Geometry check sheet. Reference: the model listing, model coordinates, mm. A direction names the side the tool comes from. Round coordinates to 2 decimals unless told otherwise and drop trailing zeros. Write each loop counter-clockwise with the first axis right and the second up, starting at its lowest first coordinate (ties: lowest second). Pieces come first, ordered by that corner, then holes. Notation, with made-up numbers: (47, -2.75) - (66, -2.75) arc R28 ccw to (66, 18.25) - close; hole circle Ø11 at (62, -39). An arc over 180 degrees is marked (long way). Return JSON: item names as keys, results as strings.
```python
from build123d import *

# Parameters (mm, degrees)
SKETCH1_W                = 15.24
SKETCH1_H                = 30.9118
BOSS_EXTRUDE1_DEPTH      = 31.115
BOSS_EXTRUDE2_DEPTH      = 6.9215
BOSS_EXTRUDE2_DEPTH_BACK = 37.9095
SKETCH2_W                = 15.24
SKETCH2_H                = 6.096
SKETCH3_R                = 5.2705
BOSS_EXTRUDE3_DEPTH      = 3.9624
SKETCH4_R                = 6.3119
BOSS_EXTRUDE4_DEPTH      = 2.5019
CUT_EXTRUDE1_REACH       = 50.11
SKETCH8_R                = 1.5621
CUT_EXTRUDE2_REACH       = 50.11
SKETCH9_R                = 1.5621
SKETCH10_R               = 3.99415
BOSS_EXTRUDE5_DEPTH      = 2.0828
SKETCH13_R               = 1.5875
CUT_EXTRUDE3_DEPTH       = 2.54


with BuildPart() as part:
    # Sketch1 → Boss-Extrude1 (new body)
    with BuildSketch(Plane(origin=(0, 0, 0), x_dir=(1, 0, 0), z_dir=(0, 1, 0))):
        with Locations((7.62, 15.4559)):
            Rectangle(SKETCH1_W, SKETCH1_H)
    extrude(amount=BOSS_EXTRUDE1_DEPTH)

    # Sketch2 → Boss-Extrude2 (add, two sides: drawn at the far end of the back side and taken through both)
    with BuildSketch(Plane.XY.offset(-BOSS_EXTRUDE2_DEPTH_BACK)):
        with Locations((7.62, 22.352)):
            Rectangle(SKETCH2_W, SKETCH2_H)
    extrude(amount=BOSS_EXTRUDE2_DEPTH + BOSS_EXTRUDE2_DEPTH_BACK)

    # Sketch3 → Boss-Extrude3 (add)
    with BuildSketch(Plane(origin=(0, 0, -30.9118), x_dir=(-1, 0, 0), z_dir=(0, 0, -1))):
        with Locations(Location((-7.62, 8.2804, 0), (0, 0, 180))):
            Circle(SKETCH3_R)
    extrude(amount=BOSS_EXTRUDE3_DEPTH)

    # Sketch4 → Boss-Extrude4 (add)
    with BuildSketch(Plane(origin=(0, 31.115, 0), x_dir=(1, 0, 0), z_dir=(0, 1, 0))):
        with Locations(Location((7.62, 24.2951, 0), (0, 0, 90))):
            Circle(SKETCH4_R)
    extrude(amount=BOSS_EXTRUDE4_DEPTH)

    # Sketch8 → Cut-Extrude1 (cut, up to next)
    with BuildSketch(Plane(origin=(0, 25.4, 0), x_dir=(1, 0, 0), z_dir=(0, 1, 0)), mode=Mode.PRIVATE) as cut_extrude1_sk1:
        with Locations(Location((7.62, -3.46075, 0), (0, 0, 270))):
            Circle(SKETCH8_R)
    cut_extrude1_tool1 = extrude(cut_extrude1_sk1.sketch, amount=-CUT_EXTRUDE1_REACH, mode=Mode.PRIVATE) & part.part
    add(cut_extrude1_tool1.solids().sort_by_distance((7.62, 25.4, 3.46075))[0], mode=Mode.SUBTRACT)

    # Sketch9 → Cut-Extrude2 (cut, up to next)
    with BuildSketch(Plane(origin=(0, 25.4, 0), x_dir=(1, 0, 0), z_dir=(0, 1, 0)), mode=Mode.PRIVATE) as cut_extrude2_sk1:
        with Locations(Location((7.62, 34.41065, 0), (0, 0, 270))):
            Circle(SKETCH9_R)
    cut_extrude2_tool1 = extrude(cut_extrude2_sk1.sketch, amount=-CUT_EXTRUDE2_REACH, mode=Mode.PRIVATE) & part.part
    add(cut_extrude2_tool1.solids().sort_by_distance((7.62, 25.4, -34.41065))[0], mode=Mode.SUBTRACT)

    # Sketch10 → Boss-Extrude5 (add)
    with BuildSketch(Plane(origin=(0, 33.6169, 0), x_dir=(1, 0, 0), z_dir=(0, 1, 0))):
        with Locations(Location((7.62, 24.2951, 0), (0, 0, 270))):
            Circle(SKETCH10_R)
    extrude(amount=BOSS_EXTRUDE5_DEPTH)

    # Sketch13 → Cut-Extrude3 (cut)
    with BuildSketch(Plane(origin=(0, 35.6997, 0), x_dir=(1, 0, 0), z_dir=(0, 1, 0))):
        with Locations(Location((7.62, 24.2951, 0), (0, 0, 270))):
            Circle(SKETCH13_R)
    extrude(amount=-CUT_EXTRUDE3_DEPTH, mode=Mode.SUBTRACT)


solid = part.part
```
(1) Access from +Z, -Z, +X, -X, +Y, -Y to the whole of each face (thin tool, end or side, straight path). Record for faces 5 (the face through (5.8, 19.304, 3.4)), 6 (the face through (8.09, 22.39, -32.92)), 7 (the face through (10.453, 3.836, -32.865)), 8 (the face through (8, 28, -30.912)).
Response values:
{"face 5": "+Z, +X, -X, -Y", "face 6": "+Y", "face 7": "-Z", "face 8": "-Z, +X, -X, +Y"}
(2) Gauge pin test, flat ends, axial feed: pin 1 (1 mm diameter, centred on x = 10.5, z = -1, fed in from +Y) (3 decimals); pin 2 (1 mm diameter, centred on x = 7, z = -23.5, fed in from +Y); pin 3 (5.5 mm diameter, centred on x = 6.5, z = 4.5, fed in from -Y); pin 4 (3 mm diameter, centred on x = 7.62, z = 3.46, fed in from -Y). Record the tip position at first contact, or that the pin passes through.
Response values:
{"pin 1": "stops at y = 31.115", "pin 2": "stops at y = 33.16", "pin 3": "stops at y = 19.3", "pin 4": "passes through"}
(3) Release check for a two-part mould opening along Y. For faces 1 (the face through (6, 35.7, -23)), 2 (the face through (8, 14, -30.912)), 3 (the face through (8, 22, 6.922)), 4 (the face through (5.8, 19.304, -34.5)) record: pulls with the +Y half, pulls with the -Y half, needs draft (parallel to the pull), parting line crosses it, or undercut.
Response values:
{"face 1": "pulls with the +Y half", "face 2": "undercut", "face 3": "needs draft", "face 4": "undercut"}
(4) Material ranges on line 1 along Z through (x, y) = (8.25, 21); line 2 along Y through (x, z) = (14.75, -34); line 3 along Z through (x, y) = (14.25, 31), recorded low to high. Write a range as [from, to].
Response values:
{"line 1": "z = [-37.91, -35.84], [-32.98, 2.03], [4.89, 6.92]", "line 2": "y = [19.3, 25.4]", "line 3": "z = [-30.91, 0]"}
(5) Section check B-B, the plane z = 4. Enter the section's corners in (x, y).
Response values:
{"outline": "(0, 19.3) - (6.15, 19.3) - (6.15, 25.4) - (0, 25.4) - close; (9.09, 19.3) - (15.24, 19.3) - (15.24, 25.4) - (9.09, 25.4) - close"}
(6) Section check C-C, the plane y = 6.5. Enter the section's corners in (x, z), plus the area to 3 significant figures.
Response values:
{"outline": "(0, -30.91) - (2.66, -30.91) - (2.66, -34.87) - (12.58, -34.87) - (12.58, -30.91) - (15.24, -30.91) - (15.24, 0) - (0, 0) - close", "area": "510 mm^2"}
(7) Section check D-D, the plane x = 7.62. Give the number of separate pieces and of enclosed holes in the cut face, plus the area to 3 significant figures.
Response values:
{"separate pieces": "3", "enclosed holes": "0", "area": "1,090 mm^2"}
(8) Section check A-A, the plane y = 24.5. Enter the section's corners in (x, z), plus the area to 3 significant figures.
Response values:
{"outline": "(0, -37.91) - (15.24, -37.91) - (15.24, 6.92) - (0, 6.92) - close; hole circle Ø3.12 at (7.62, -34.41); hole circle Ø3.12 at (7.62, 3.46)", "area": "668 mm^2"}
